Could you check a few things on this drawing? It's one solid part, dimensions in mm from its lowest x, y, z. Give positions to 0.01 mm unless a question says otherwise; leave off trailing zeros. Loops run counter-clockwise (first coordinate to the right, second up) from the corner with the lowest first, then second, coordinate; pieces in that order, holes last. Notation, with made-up numbers: (-12.5, 39) - (1.5, 39) arc R11 ccw to (1.5, 43) - close; hole circle Ø10 at (68.25, 86.5). An arc over 180 degrees is marked (long way). Put each result on its own line as item: value. Start each with the question number.
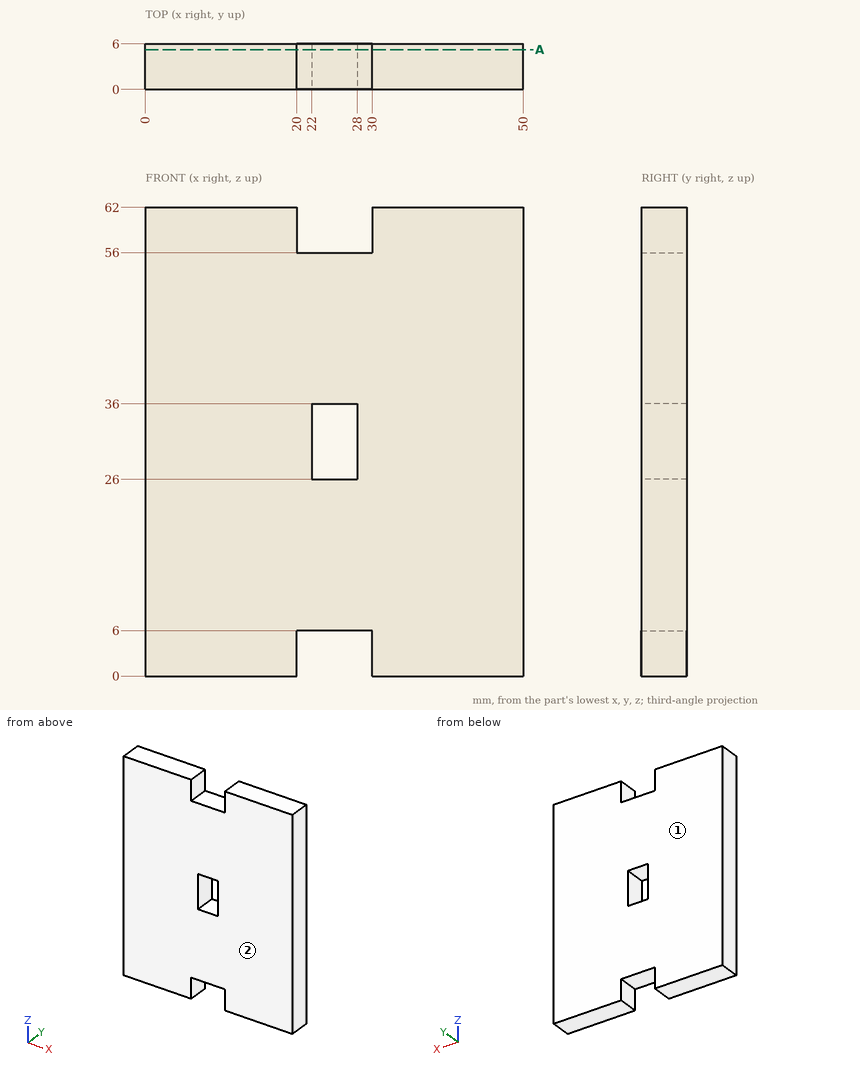
1) I need wall thicknesses on line 1 (X direction, y = 4.25, z = 30); line 2 (X direction, y = 3, z = 4.5). Which ranges of each line are inside material? Lowest first, please.
2) I'm going to push a flat-ended pin straight in: P1, Ø3, axis at x = 26, y = 4, coming from the +Z side. Where does the tip first touch, or does it pass through?
3) Suppose I cut it at A-A on y = 5.25. Please give me the cut outline in (x, z).
4) Thinking about a two-plate mould opening in Y: for the marked faces 1 and 2, which applies, pulls with the +Y half, pulls with the -Y half, needs draft (parallel to the pull), parting line crosses it, or undercut?
Ans:
1. line 1: x = 0 to 22, 28 to 50
1. line 2: x = 0 to 20, 30 to 50
2. P1: stops at z = 56
3. outline: (0, 0) - (20, 0) - (20, 6) - (30, 6) - (30, 0) - (50, 0) - (50, 62) - (30, 62) - (30, 56) - (20, 56) - (20, 62) - (0, 62) - close; hole (22, 26) - (28, 26) - (28, 36) - (22, 36) - close
4. face 1: pulls with the +Y half
4. face 2: pulls with the -Y half
